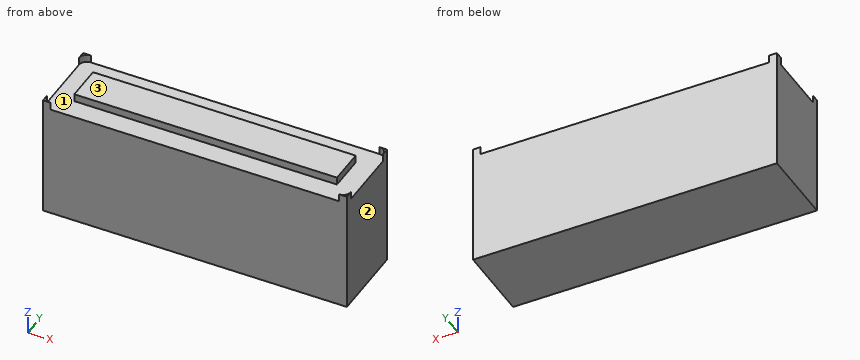
from build123d import *

# Parameters (mm, degrees)
F1_DEPTH = 76.2
F2_W     = 161.925
F2_H     = 22.225
F3_DEPTH = 4.7625


with BuildPart() as f1:
    # F0 (on Top) → F1 (new body)
    with BuildSketch(Plane.XY):
        Polygon((0, 0), (4.7625, 0), (182.5625, 0), (187.325, 0), (187.325, 4.7625), (187.325, 42.8625), (187.325, 47.625), (182.5625, 47.625), (4.7625, 47.625), (0, 47.625), (0, 42.8625), (0, 4.7625), align=None)
    extrude(amount=-F1_DEPTH)

    # F2 (on face) → F3 (cut)
    with BuildSketch(Plane.XY):
        with BuildLine():
            Line((187.325, 4.7625), (187.325, 42.8625))
            ThreePointArc((187.325, 42.8625), (185.930096, 46.230096), (182.5625, 47.625))
            Line((182.5625, 47.625), (4.7625, 47.625))
            ThreePointArc((4.7625, 47.625), (1.394904, 46.230096), (0, 42.8625))
            Line((0, 42.8625), (0, 4.7625))
            ThreePointArc((0, 4.7625), (1.394904, 1.394904), (4.7625, 0))
            Line((4.7625, 0), (182.5625, 0))
            ThreePointArc((182.5625, 0), (185.930096, 1.394904), (187.325, 4.7625))
        make_face()
        with Locations((93.6625, 23.8125)):
            Rectangle(F2_W, F2_H, mode=Mode.SUBTRACT)
    extrude(amount=-F3_DEPTH, mode=Mode.SUBTRACT)


solid = f1.part
Read the model definition and answer for the solid it produces. Units are mm, in the model's axes. Face numbers are marked on the shaded views. Give positions to 0.01 mm unless a question says otherwise; leave off trailing zeros. Write each loop counter-clockwise with the first axis right and the second up, starting at its lowest first coordinate (ties: lowest second). Pieces come first, ordered by that corner, then holes. Notation, with made-up numbers: (45.25, -17.75) -> (53.25, -17.75) arc R16 cw to (53.25, 4.25) -> close; hole circle Ø9 at (48.5, 30). An arc over 180 degrees is marked (long way). Answer as a JSON object with one key per item and string values. Group by question number.
1) Find section B-B (y = 7). Write down the section's boundary in (x, z) (1 decimal), and give its area (3 significant figures).
2) Each of these flat-tipped pins is pushed along its axis until it touches: P1, Ø4, axis at y = 20.5, z = -1.5, coming from the -X side; P2, Ø1.4, axis at x = 56, z = -1.5, coming from the +Y side (3 decimals); P3, Ø2.5, axis at y = 29.5, z = -2.5, coming from the +X side (3 decimals). Where does it stop, or does it pass through?
3) Consider L1, parallel to Z at x = 28.5, y = 9. Determine where the line is inside the solid, lowest interval first. Write a range as from..to.
4) Find section A-A (x = 48). Write down the section's boundary in (y, z) (1 decimal), and give its area (3 significant figures).
5) The mould has two halves that part along X. Classify the marked faces 1, 2 and 3: +X half, -X half, draft (parallel to the pull), parting line (faces both ways), or undercut.
Values follow:
{
 "1": {"outline": "(0, -76.2) -> (187.3, -76.2) -> (187.3, -4.8) -> (0, -4.8) -> close", "area": "13,400 mm2"},
 "2": {"P1": "stops at x = 12.7", "P2": "stops at y = 34.925", "P3": "stops at x = 174.625"},
 "3": {"L1": "z = -76.2..-4.76"},
 "4": {"outline": "(0, -76.2) -> (47.6, -76.2) -> (47.6, -4.8) -> (34.9, -4.8) -> (34.9, 0) -> (12.7, 0) -> (12.7, -4.8) -> (0, -4.8) -> close", "area": "3,510 mm2"},
 "5": {"face 1": "undercut", "face 2": "+X half", "face 3": "draft"}
}
